Verification items for the finished model (mm, model axes). Face numbers are marked on the shaded views. A direction names the side the tool comes from. Give positions to 0.01 mm unless a question says otherwise; leave off trailing zeros. Order: outer loops, then holes, each group sorted by start corner. A loop starts at its lowest first (then second) coordinate and runs counter-clockwise, first axis right, second up.
(1) Sectioned sample at B-B on z = 0. Record the cut outline in (x, y), plus the area to 3 significant figures.
(2) Sectioned sample at C-C on y = 6.5. Record the cut outline in (x, z), plus the area to 3 significant figures.
(3) Mould release check, pull along X, two halves, no side actions. Record for the marked faces 1, 2, 3 and 4: pulls with the +X half, pulls with the -X half, needs draft (parallel to the pull), parting line crosses it, or undercut.
(4) Sectioned sample at D-D on y = -1.25. Record the cut outline in (x, z), plus the area to 3 significant figures.
(5) Scan lines: L1, parallel to Z at x = 0, y = -2.25; L2, parallel to Z at x = 0, y = 10. Record each from-to range of solid material in increasing order.
(6) Access from +Z, -Z, +X, -X, +Y, -Y to the whole of each face (thin tool, end or side, straight path). Record for the marked faces 5 and 6.
(7) Sectioned sample at A-A on x = 0. Record the cut outline in (y, z), plus the area to 3 significant figures.
(8) Gauge pin test, flat ends, axial feed: pin 1 (6 mm diameter, centred on y = -5, z = -5.5, fed in from -X); pin 2 (1 mm diameter, centred on x = 8, y = -2.5, fed in from -Z); pin 3 (1 mm diameter, centred on x = -1, z = 5.5, fed in from -Y). Record the tip position at first contact, or that the pin passes through.
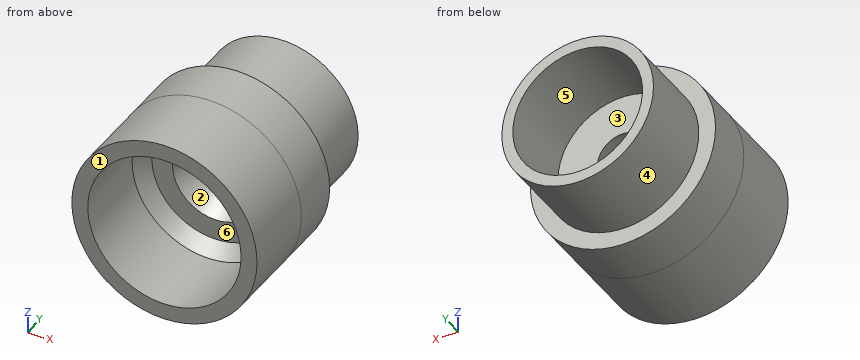
```python
from build123d import *

# Parameters (mm, degrees)
CROQUIS1_R              = 11.05
CROQUIS1_R_2            = 9.05
SALIENTE_EXTRUIR1_DEPTH = 9.4
CROQUIS2_R              = 11.05
SALIENTE_EXTRUIR2_DEPTH = 6
CROQUIS3_R              = 9.05
CROQUIS3_R_2            = 7.74
SALIENTE_EXTRUIR3_DEPTH = 9.6
CROQUIS4_R              = 3.05
CORTAR_EXTRUIR1_DEPTH   = 9.6
CROQUIS5_R              = 9.15
CORTAR_EXTRUIR2_DEPTH   = 9.4


with BuildPart() as part:
    # Croquis1 → Saliente-Extruir1 (new body)
    with BuildSketch(Plane(origin=(0, 0, 0), x_dir=(1, 0, 0), z_dir=(0, 1, 0))):
        Circle(CROQUIS1_R)
        Circle(CROQUIS1_R_2, mode=Mode.SUBTRACT)
    extrude(amount=-SALIENTE_EXTRUIR1_DEPTH)

    # Croquis2 → Saliente-Extruir2 (add)
    with BuildSketch(Plane(origin=(0, 0, 0), x_dir=(1, 0, 0), z_dir=(0, 1, 0))):
        Circle(CROQUIS2_R)
    extrude(amount=SALIENTE_EXTRUIR2_DEPTH)

    # Croquis3 → Saliente-Extruir3 (add)
    with BuildSketch(Plane(origin=(0, 6, 0), x_dir=(1, 0, 0), z_dir=(0, 1, 0))):
        Circle(CROQUIS3_R)
        Circle(CROQUIS3_R_2, mode=Mode.SUBTRACT)
    extrude(amount=SALIENTE_EXTRUIR3_DEPTH)

    # Croquis4 → Cortar-Extruir1 (cut)
    with BuildSketch(Plane(origin=(0, 6, 0), x_dir=(1, 0, 0), z_dir=(0, 1, 0))):
        Circle(CROQUIS4_R)
    extrude(amount=-CORTAR_EXTRUIR1_DEPTH, mode=Mode.SUBTRACT)

    # Croquis5 → Cortar-Extruir2 (cut)
    with BuildSketch(Plane.XZ.offset(9.4)):
        Circle(CROQUIS5_R)
    extrude(amount=-CORTAR_EXTRUIR2_DEPTH, mode=Mode.SUBTRACT)

    # Croquis6 → Cortar-Revolución1 (revolve, cut)
    with BuildSketch(Plane.XY):
        Polygon((-9.15, 0), (-7.643411501, 1.506588499), (-5.172223625, 1.506588499), (-3.05, 6), (0, 6), (0, 1.506588499), (0, 0), align=None)
    revolve(axis=Axis((0, 1.506588499, 0), (0, -1, 0)), mode=Mode.SUBTRACT)


solid = part.part
```
Ans:
1. outline: (-11.05, -9.4) - (-9.15, -9.4) - (-9.15, 0) - (-7.64, 1.51) - (-5.17, 1.51) - (-3.05, 6) - (-7.74, 6) - (-7.74, 15.6) - (-9.05, 15.6) - (-9.05, 6) - (-11.05, 6) - close; (3.05, 6) - (5.17, 1.51) - (7.64, 1.51) - (9.15, 0) - (9.15, -9.4) - (11.05, -9.4) - (11.05, 6) - (9.05, 6) - (9.05, 15.6) - (7.74, 15.6) - (7.74, 6) - close
1. area: 131 mm2
2. outline: circle Ø18.1 at (0, 0); hole circle Ø15.48 at (0, 0)
2. area: 69.1 mm2
3. face 1: needs draft
3. face 2: undercut
3. face 3: undercut
3. face 4: parting line crosses it
4. outline: circle Ø22.1 at (0, 0); hole circle Ø18.3 at (0, 0)
4. area: 121 mm2
5. L1: z = -11.05 to -9.15, 9.15 to 11.05
5. L2: z = -9.05 to -7.74, 7.74 to 9.05
6. face 5: +Y
6. face 6: -Y
7. outline: (-9.4, -11.05) - (6, -11.05) - (6, -9.05) - (15.6, -9.05) - (15.6, -7.74) - (6, -7.74) - (6, -3.05) - (1.51, -5.17) - (1.51, -7.64) - (0, -9.15) - (-9.4, -9.15) - close; (-9.4, 9.15) - (0, 9.15) - (1.51, 7.64) - (1.51, 5.17) - (6, 3.05) - (6, 7.74) - (15.6, 7.74) - (15.6, 9.05) - (6, 9.05) - (6, 11.05) - (-9.4, 11.05) - close
7. area: 131 mm2
8. pin 1: stops at x = -10.76
8. pin 2: stops at z = -8.11
8. pin 3: stops at y = 1.51
